Could you check a few things on this model? Use its own coordinates, in mm. A direction names the side the tool comes from. Coordinates: 2 decimals unless noted, no trailing zeros. Write each loop counter-clockwise with the first axis right and the second up, starting at its lowest first coordinate (ties: lowest second). Pieces come first, ordered by that corner, then holes. Notation, with made-up numbers: (75, 54.5) - (119, 54.5) arc R20 cw to (119, 63.5) - close; hole circle Ø8 at (64.25, -34). An arc over 180 degrees is marked (long way). Answer as a JSON object with one key per item and string values. Group by question number.
1) If we section it at B-B (x = 0): Write out the boundary of the cut face in (y, z).
2) We'd pull the mould along Y, two halves only. Please class faces 6 (the flat face through (-15, -18, -97)), 7 (the flat face through (-0.2, -15.5, -94)), 8 (the flat face through (0, 0, 2)): released by +Y, released by -Y, zero draft, split by the parting line, or undercut.
3) If we section it at D-D (x = -9.5): Write out the boundary of the cut face in (y, z).
4) If we section it at C-C (y = -21): Write out the boundary of the cut face in (x, z), plus the area to 3 significant figures.
5) Please list where these lines run through material, in increasing order: line 1 along Z through (x, y) = (-3, -14); line 2 along Y through (x, z) = (22.5, 15); line 3 along Y through (x, z) = (-3, 20.5).
6) If we section it at A-A (z = 17): Write out the boundary of the cut face in (x, y), plus the area to 3 significant figures.
7) On a 3-axis mill with a long thin cutter (end or side, diameter ignored), from which of +Z, -Z, +X, -X, +Y, -Y can I reach the whole of each face in a straight line? I mean faces 1 (the cylindrical face through (-1.08, -16.12, 1.32)), 2 (the flat face through (15, -18, 97)), 3 (the flat face through (0, -18, 100)), 4 (the flat face through (0, -18, -100)), 5 (the flat face through (-15, -18, 97)). Say none if no direction works.
8) Will these pins go through, and if not, where does the flat tip stop? pin 1 Ø10 at (x, y) = (14, -12) entering from -Z; pin 2 Ø5 at (y, z) = (-18.5, 98) entering from +X; pin 3 Ø1.5 at (x, z) = (-14.5, -48) entering from -Y.
```python
from build123d import *

# Parameters (mm, degrees)
F0_W     = 50
F0_H     = 250
F1_DEPTH = 6
F2_W     = 30
F2_H     = 6
F3_DEPTH = 25
F4_R     = 5
F5_DEPTH = 188


with BuildPart() as f1:
    # F0 (on Front) → F1 (new body)
    with BuildSketch(Plane.XZ):
        Rectangle(F0_W, F0_H)
    extrude(amount=F1_DEPTH)

    # F2 (on face) → F3 (join)
    with BuildSketch(Plane.XZ.offset(6)):
        with Locations((0, 97)):
            Rectangle(F2_W, F2_H)
        with Locations((0, -97)):
            Rectangle(F2_W, F2_H)
    extrude(amount=F3_DEPTH)

    # F4 (on face) → F5 (join, through all)
    with BuildSketch(Plane(origin=(0, 0, 94), x_dir=(1, 0, 0), z_dir=(0, 0, -1))):
        with Locations((0, 21)):
            Circle(F4_R)
    extrude(amount=F5_DEPTH)


solid = f1.part
```
Here are the results:
{
 "1": {"outline": "(-31, -100) - (-6, -100) - (-6, -125) - (0, -125) - (0, 125) - (-6, 125) - (-6, 100) - (-31, 100) - (-31, 94) - (-26, 94) - (-26, -94) - (-31, -94) - close; hole (-16, -94) - (-6, -94) - (-6, 94) - (-16, 94) - close"},
 "2": {"face 6": "zero draft", "face 7": "undercut", "face 8": "released by +Y"},
 "3": {"outline": "(-31, -100) - (-6, -100) - (-6, -125) - (0, -125) - (0, 125) - (-6, 125) - (-6, 100) - (-31, 100) - (-31, 94) - (-6, 94) - (-6, -94) - (-31, -94) - close"},
 "4": {"outline": "(-15, -100) - (15, -100) - (15, -94) - (5, -94) - (5, 94) - (15, 94) - (15, 100) - (-15, 100) - (-15, 94) - (-5, 94) - (-5, -94) - (-15, -94) - close", "area": "2,240 mm²"},
 "5": {"line 1": "z = -100 to -94, 94 to 100", "line 2": "y = -6 to 0", "line 3": "y = -25 to -17, -6 to 0"},
 "6": {"outline": "(-25, -6) - (25, -6) - (25, 0) - (-25, 0) - close; circle Ø10 at (0, -21)", "area": "379 mm²"},
 "7": {"face 1": "none", "face 2": "+Z, -Z, +X, -Y", "face 3": "+Z, +X, -X, -Y", "face 4": "-Z, +X, -X, -Y", "face 5": "+Z, -Z, -X, -Y"},
 "8": {"pin 1": "stops at z = -100", "pin 2": "stops at x = 15", "pin 3": "stops at y = -6"}
}
